CAD build for the part. Positions are in the model's coordinates, mm. Round coordinates to 2 decimals unless told otherwise and drop trailing zeros. Order: outer loops, then holes, each group sorted by start corner. A loop starts at its lowest first (then second) coordinate and runs counter-clockwise, first axis right, second up. Notation, with made-up numbers: M 77,7.25 L 125,7.25 A20 cw 125,16.25 Z; hole C 24.5,3.25 d4. An arc over 180 degrees is marked long. Put each result on its own line as item: value.
Autodesk Inventor part; units mm, degrees
ref_plane "YZ Plane" through (0, 0, 0) normal (1, 0, 0) x (0, 1, 0)
ref_plane "XZ Plane" through (0, 0, 0) normal (0, 1, 0) x (-1, 0, 0)
ref_plane "XY Plane" through (0, 0, 0) normal (0, 0, 1) x (1, 0, 0)
sketch "Sketch1" plane through (0, 0, 0) normal (0, 1, 0) x (-1, 0, 0)
  circle A0 centre (-2.8921, -102.8959) radius 2.1844
  circle A1 centre (22.5079, -102.8959) radius 2.1844
  circle A2 centre (-2.8921, 113.0041) radius 2.1844
  circle A3 centre (22.5079, 113.0041) radius 2.1844
  arc A4 (28.8579, 113.0041) -> (22.5079, 119.3541) centre (22.5079, 113.0041) ccw
  arc A5 (-2.8921, 119.3541) -> (-6.7021, 118.0841) centre (-2.8921, 113.0041) ccw
  arc A6 (-6.7021, -107.9759) -> (-2.8921, -109.2459) centre (-2.8921, -102.8959) ccw
  arc A7 (22.5079, -109.2459) -> (28.8579, -102.8959) centre (22.5079, -102.8959) ccw
  line L0 (-2.8921, 119.3541) -> (22.5079, 119.3541)
  line L1 (28.8579, 113.0041) -> (28.8579, -102.8959)
  line L2 (22.5079, -109.2459) -> (-2.8921, -109.2459)
  line L3 (-16.8621, 110.4641) -> (-6.7021, 118.0841)
  line L4 (-16.8621, -100.3559) -> (-6.7021, -107.9759)
  line L5 (-21.9421, 100.3041) -> (-21.9421, -90.1959)
  arc A8 (-16.8621, 110.4641) -> (-21.9421, 100.3041) centre (-9.2421, 100.3041) ccw
  arc A9 (-21.9421, -90.1959) -> (-16.8621, -100.3559) centre (-9.2421, -90.1959) ccw
  line L6 (-2.8921, 119.3541) -> (22.5079, 119.3541)
  line L7 (22.5079, -109.2459) -> (-2.8921, -109.2459)
  line L8 (28.8579, 113.0041) -> (28.8579, -102.8959)
  point P0 (0, 0)
  dimension "d0" = 12.7
  dimension "d1" = 12.7
  dimension "d2" = 12.7
  dimension "d3" = 12.7
extrude "Extrusion1" add sketch "Sketch1" along normal blind 1.5875
properties part number "Wedge" material "Acetal Resin, White"
Item 1: Mould opens along Z. For faces 1 (the cylindrical face through (-26.95, 0.78, 117.54)), 2 (the cylindrical face through (20.564, 0.783, -95.949)), 3 (the cylindrical face through (-24.526, 0.783, 113.841)), 4 (the cylindrical face through (1.72, 0.78, -104.74)) say: pulls with the +Z half, pulls with the -Z half, needs draft (parallel to the pull), parting line crosses it, or undercut.
Answers below:
face 1: pulls with the +Z half
face 2: pulls with the -Z half
face 3: undercut
face 4: undercut
Item 2: Probe line 1 along Z through (x, y) = (2, 1.2); line 2 along Z through (x, y) = (4.5, 0.55); line 3 along X through (y, z) = (0.5, -99.5). List the from-to ranges inside material, lowest first. Write a range as [from, to].
Answers below:
line 1: [-109.25, -104.89], [-100.9, 111.01], [115, 119.35]
line 2: [-109.04, -104.37], [-101.42, 111.53], [114.48, 119.15]
line 3: [-28.86, 17.89]
Item 3: Band-saw the part on B-B on x = 11. Give the cut face in (y, z).
Answers below:
outline: M 0,-104.75 L 1.59,-104.75 L 1.59,114.86 L 0,114.86 Z
Item 4: Band-saw the part on A-A on y = 0.85. Give the cut face in (x, z), and give its area (3 significant figures).
Answers below:
outline: M -28.86,-102.9 A6.35 ccw -22.51,-109.25 L 2.89,-109.25 A6.35 ccw 6.7,-107.98 L 16.86,-100.36 A12.7 ccw 21.94,-90.2 L 21.94,100.3 A12.7 ccw 16.86,110.46 L 6.7,118.08 A6.35 ccw 2.89,119.35 L -22.51,119.35 A6.35 ccw -28.86,113 Z; hole C -22.51,-102.9 d4.37; hole C -22.51,113 d4.37; hole C 2.89,-102.9 d4.37; hole C 2.89,113 d4.37
area: 11,300 mm²
Item 5: Pin check, flat tips, straight feed: P1, Ø3.5, axis at x = 2.89, z = -102.9, coming from the +Y side; P2, Ø1, axis at x = -16, z = -71.5, coming from the -Y side. Stop position of each tip, or through.
Answers below:
P1: through
P2: y = 0
